Build history of the part. All positions in model axes, mm. Face numbers are marked on the shaded views. A direction names the side the tool comes from. Coordinates: 2 decimals unless noted, no trailing zeros.
(1) Flat gauge pins, fed straight in: P1, Ø0.7, axis at x = 22, z = 0.5, coming from the +Y side (3 decimals); P2, Ø5, axis at x = 33, z = -1, coming from the +Y side (3 decimals); P3, Ø1.7, axis at x = -7.5, y = -2.5, coming from the -Z side. Where does each tip first touch, or does it go through?
(2) Tool access for the marked faces 1, 2 and 3: list every direction of +Z, -Z, +X, -X, +Y, -Y with a clear straight run to the whole face (end or side of a thin tool).
(3) Two-plate mould, pull along Z, no slides. Class the marked faces 4, 5 and 6: pulls with the +Z half, pulls with the -Z half, needs draft (parallel to the pull), parting line crosses it, or undercut.
(4) Wall check: L1, parallel to Z at x = 22, y = 3.25; L2, parallel to Z at x = -2, y = -0.5; L3, parallel to X at y = 3, z = -1.5. Give the ranges that are in metal, low to high.
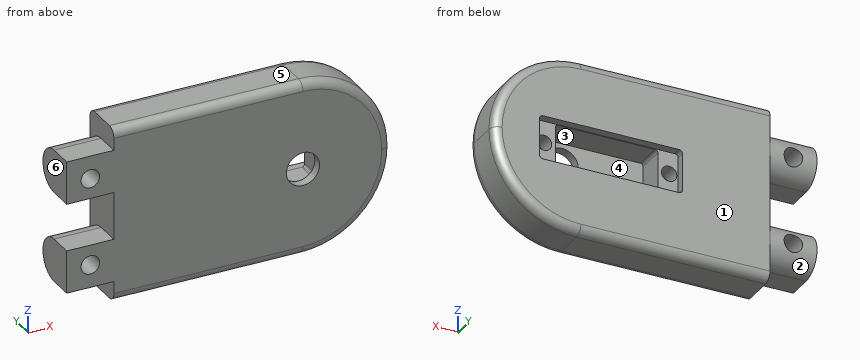
from build123d import *

# Parameters (mm, degrees)
SKETCH1_W           = 40
SKETCH1_H           = 10.610001376
BOSS_EXTRUDE1_DEPTH = 63.235
CUT_EXTRUDE1_DEPTH  = 11.610001375
CUT_EXTRUDE2_DEPTH  = 1.95
CUT_EXTRUDE3_DEPTH  = 6.56
SKETCH5_R           = 3.8
CUT_EXTRUDE4_DEPTH  = 3.100001375
SKETCH6_R           = 1.75
CUT_EXTRUDE5_DEPTH  = 4.1
SKETCH7_R           = 1.125
CUT_EXTRUDE6_DEPTH  = 2
FILLET1_R           = 2
BOSS_EXTRUDE2_DEPTH = 10.77
SKETCH9_R           = 2.125
CUT_EXTRUDE7_DEPTH  = 11.610001375


with BuildPart() as part:
    # Sketch1 → Boss-Extrude1 (new body)
    with BuildSketch(Plane(origin=(0, 0, 0), x_dir=(0, 0, -1), z_dir=(1, 0, 0))):
        Rectangle(SKETCH1_W, SKETCH1_H)
    extrude(amount=BOSS_EXTRUDE1_DEPTH)

    # Sketch2 → Cut-Extrude1 (cut, through all)
    with BuildSketch(Plane(origin=(0, 5.305000688, 0), x_dir=(1, 0, 0), z_dir=(0, 1, 0))):
        with BuildLine():
            Line((63.235, -20), (63.235, 0))
            ThreePointArc((63.235, 0), (57.377135624, -14.142135624), (43.235, -20))
            Line((43.235, -20), (63.235, -20))
        make_face()
    cut_extrude1 = extrude(amount=-CUT_EXTRUDE1_DEPTH, mode=Mode.SUBTRACT)

    # Mirror1: Cut-Extrude1 across plane
    add(cut_extrude1.mirror(Plane.XY), mode=Mode.SUBTRACT)

    # Sketch3 → Cut-Extrude2 (cut)
    with BuildSketch(Plane(origin=(0, 5.305000688, 0), x_dir=(1, 0, 0), z_dir=(0, 1, 0))):
        with BuildLine():
            Line((20, 4.2), (20, -4.2))
            ThreePointArc((20, -4.2), (20.234314575, -4.765685425), (20.8, -5))
            Line((20.8, -5), (31.17, -5))
            Line((31.17, -5), (41.54, -5))
            Line((41.54, -5), (51.91, -5))
            ThreePointArc((51.91, -5), (52.475685425, -4.765685425), (52.71, -4.2))
            Line((52.71, -4.2), (52.71, 4.2))
            ThreePointArc((52.71, 4.2), (52.475685425, 4.765685425), (51.91, 5))
            Line((51.91, 5), (41.54, 5))
            Line((41.54, 5), (31.17, 5))
            Line((31.17, 5), (20.8, 5))
            ThreePointArc((20.8, 5), (20.234314575, 4.765685425), (20, 4.2))
        make_face()
    extrude(amount=-CUT_EXTRUDE2_DEPTH, mode=Mode.SUBTRACT)

    # Sketch4 → Cut-Extrude3 (cut)
    with BuildSketch(Plane(origin=(0, 3.355000688, 0), x_dir=(1, 0, 0), z_dir=(0, 1, 0))):
        with BuildLine():
            Line((48.07, -4.2), (48.07, 4.2))
            ThreePointArc((48.07, 4.2), (47.968188406, 4.549269911), (47.694647782, 4.78912528))
            ThreePointArc((47.694647782, 4.78912528), (47.560656617, 4.834598862), (47.42, 4.85))
            Line((47.42, 4.85), (25.29, 4.85))
            ThreePointArc((25.29, 4.85), (24.830380592, 4.659619408), (24.64, 4.2))
            Line((24.64, 4.2), (24.64, -4.2))
            ThreePointArc((24.64, -4.2), (24.830380592, -4.659619408), (25.29, -4.85))
            Line((25.29, -4.85), (47.42, -4.85))
            ThreePointArc((47.42, -4.85), (47.749899473, -4.760059227), (47.988502289, -4.515127192))
            ThreePointArc((47.988502289, -4.515127192), (48.049295832, -4.362747522), (48.07, -4.2))
        make_face()
    extrude(amount=-CUT_EXTRUDE3_DEPTH, mode=Mode.SUBTRACT)

    # Sketch5 → Cut-Extrude4 (cut, through all)
    with BuildSketch(Plane(origin=(0, -3.204999312, 0), x_dir=(1, 0, 0), z_dir=(0, 1, 0))):
        with Locations((43.235, 0)):
            Circle(SKETCH5_R)
    extrude(amount=-CUT_EXTRUDE4_DEPTH, mode=Mode.SUBTRACT)

    # Sketch6 → Cut-Extrude5 (cut)
    with BuildSketch(Plane(origin=(0, 3.355000688, 0), x_dir=(1, 0, 0), z_dir=(0, 1, 0))):
        with Locations((50.655, 0)):
            Circle(SKETCH6_R)
        with Locations((22.055, 0)):
            Circle(SKETCH6_R)
    extrude(amount=-CUT_EXTRUDE5_DEPTH, mode=Mode.SUBTRACT)

    # Sketch7 → Cut-Extrude6 (cut)
    with BuildSketch(Plane(origin=(0, -0.744999312, 0), x_dir=(1, 0, 0), z_dir=(0, 1, 0))):
        with Locations((50.655, 0)):
            Circle(SKETCH7_R)
        with Locations((22.055, 0)):
            Circle(SKETCH7_R)
    extrude(amount=-CUT_EXTRUDE6_DEPTH, mode=Mode.SUBTRACT)

    # Fillet1
    fillet1_edges = [part.edges().sort_by_distance(p)[0] for p in [
        (21.6175, 5.305000688, 20),
        (21.6175, -5.305000688, 20),
        (63.235, -5.305000688, 0),
        (63.235, 5.305000688, 0),
        (21.6175, 5.305000688, -20),
        (21.6175, -5.305000688, -20),
    ]]
    fillet(fillet1_edges, radius=FILLET1_R)

    # Sketch8 → Boss-Extrude2 (add)
    with BuildSketch(Plane.ZY):
        with BuildLine():
            Line((-15.221247138, 0.365000688), (-15.221247138, -5.305000688))
            Line((-15.221247138, -5.305000688), (-5.421247138, -5.305000688))
            Line((-5.421247138, -5.305000688), (-5.421247138, 0.365000688))
            ThreePointArc((-5.421247138, 0.365000688), (-10.321247138, 5.265000688), (-15.221247138, 0.365000688))
        make_face()
        with BuildLine():
            Line((15.221247138, 0.365000688), (15.221247138, -5.305000688))
            Line((15.221247138, -5.305000688), (5.421247138, -5.305000688))
            Line((5.421247138, -5.305000688), (5.421247138, 0.365000688))
            ThreePointArc((5.421247138, 0.365000688), (10.321247138, 5.265000688), (15.221247138, 0.365000688))
        make_face()
    extrude(amount=BOSS_EXTRUDE2_DEPTH)

    # Sketch9 → Cut-Extrude7 (cut, through all)
    with BuildSketch(Plane.XZ.offset(5.305000688)):
        with Locations((-5.385, 10)):
            Circle(SKETCH9_R)
        with Locations((-5.385, -10)):
            Circle(SKETCH9_R)
    extrude(amount=-CUT_EXTRUDE7_DEPTH, mode=Mode.SUBTRACT)


solid = part.part
Response values:
1. P1: stops at y = -2.745
1. P2: stops at y = -3.205
1. P3: stops at z = -15.22
2. face 1: +Z, -Z, +X, -X, +Y
2. face 2: -X, +Y
2. face 3: +Y
3. face 4: undercut
3. face 5: pulls with the +Z half
3. face 6: needs draft
4. L1: z = -20 to -1.75, 1.75 to 20
4. L2: z = -15.22 to -5.42, 5.42 to 15.22
4. L3: x = 0 to 21.15, 22.96 to 24.64, 48.07 to 49.75, 51.56 to 63.18
